Build history of the part. All positions in model axes, mm. A direction names the side the tool comes from. Round coordinates to 2 decimals unless told otherwise and drop trailing zeros. Order: outer loops, then holes, each group sorted by start corner. A loop starts at its lowest first (then second) coordinate and runs counter-clockwise, first axis right, second up. Notation, with made-up numbers: (79, 4.25) - (125, 4.25) arc R17 ccw to (125, 26.25) - close; hole circle Ø2 at (-34.5, -38.75). An arc over 180 degrees is marked (long way). Write each question's results on one line, items separated by ' | '. Start each with the question number.
```python
from build123d import *

# Parameters (mm, degrees)
BOSS_EXTRUDE1_DEPTH = 30
CUT_EXTRUDE3_DEPTH  = 28
SKETCH5_R           = 7.5
CUT_EXTRUDE5_DEPTH  = 4


with BuildPart() as part:
    # Sketch1 → Boss-Extrude1 (new body)
    with BuildSketch(Plane(origin=(0, 0, 0), x_dir=(1, 0, 0), z_dir=(0, 1, 0))):
        with BuildLine():
            Line((5, 0), (70, 0))
            ThreePointArc((70, 0), (73.535533906, 1.464466094), (75, 5))
            Line((75, 5), (75, 85))
            ThreePointArc((75, 85), (73.535533906, 88.535533906), (70, 90))
            Line((70, 90), (5, 90))
            ThreePointArc((5, 90), (1.464466094, 88.535533906), (0, 85))
            Line((0, 85), (0, 5))
            ThreePointArc((0, 5), (1.464466094, 1.464466094), (5, 0))
        make_face()
    extrude(amount=BOSS_EXTRUDE1_DEPTH)

    # Sketch3 → Cut-Extrude3 (cut)
    with BuildSketch(Plane(origin=(0, 0, 0), x_dir=(-1, 0, 0), z_dir=(0, -1, 0))):
        with BuildLine():
            Line((-7.5, 2.5), (-67.5, 2.5))
            ThreePointArc((-67.5, 2.5), (-71.035533906, 3.964466094), (-72.5, 7.5))
            Line((-72.5, 7.5), (-72.5, 82.5))
            ThreePointArc((-72.5, 82.5), (-71.035533906, 86.035533906), (-67.5, 87.5))
            Line((-67.5, 87.5), (-7.5, 87.5))
            ThreePointArc((-7.5, 87.5), (-3.964466094, 86.035533906), (-2.5, 82.5))
            Line((-2.5, 82.5), (-2.5, 7.5))
            ThreePointArc((-2.5, 7.5), (-3.964466094, 3.964466094), (-7.5, 2.5))
        make_face()
    extrude(amount=-CUT_EXTRUDE3_DEPTH, mode=Mode.SUBTRACT)

    # Sketch5 → Cut-Extrude5 (cut)
    with BuildSketch(Plane(origin=(75, 0, 0), x_dir=(0, 0, -1), z_dir=(1, 0, 0))):
        with Locations((35, 15)):
            Circle(SKETCH5_R)
    extrude(amount=-CUT_EXTRUDE5_DEPTH, mode=Mode.SUBTRACT)


solid = part.part
```
1. Wall check: line 1 (X direction, y = 16.75, z = -67); line 2 (Z direction, x = 62, y = 8.25); line 3 (Y direction, x = 73.6, z = -35). Give the ranges that are in metal, low to high. Write a range as from..to.
2. Cut at C-C (x = 61.5). List the corners of the cut face in (y, z), plus the area to 3 significant figures.
3. Cut at B-B (y = 15). List the corners of the cut face in (x, z), plus the area to 4 significant figures.
4. Cut at A-A (z = -35). List the corners of the cut face in (x, y), plus the area to 4 significant figures.
5. Mould opens along X. For faces 4 (the face through (1, 15, -2)), 5 (the face through (71, 13.8, -3.93)), 6 (the face through (73, 15, -1)) say: pulls with the +X half, pulls with the -X half, needs draft (parallel to the pull), parting line crosses it, or undercut.
6. 3-axis set-ups, long thin cutter, end or side, ignore diameter. For faces 1 (the face through (37, 15, 0)), 2 (the face through (37, 14, -2.5)), 3 (the face through (73.8, 20.1, -29.5)): which of +Z, -Z, +X, -X, +Y, -Y reach the whole face in a straight line?
7. Cut at D-D (z = -64.5). List the corners of the cut face in (x, y), plus the area to 3 significant figures.
8. Flat gauge pin, fed straight in: pin 1 Ø6 at (x, z) = (40, -45.5) entering from -Y. Where does the tip first touch, or does it go through?
A:
1) line 1: x = 0..2.5, 72.5..75 | line 2: z = -90..-87.5, -2.5..0 | line 3: y = 0..7.5, 22.5..30
2) outline: (0, -90) - (30, -90) - (30, 0) - (0, 0) - (0, -2.5) - (28, -2.5) - (28, -87.5) - (0, -87.5) - close | area: 320 mm^2
3) outline: (0, -85) arc R5 ccw to (5, -90) - (70, -90) arc R5 ccw to (75, -85) - (75, -42.5) - (72.5, -42.5) - (72.5, -82.5) arc R5 cw to (67.5, -87.5) - (7.5, -87.5) arc R5 cw to (2.5, -82.5) - (2.5, -7.5) arc R5 cw to (7.5, -2.5) - (67.5, -2.5) arc R5 cw to (72.5, -7.5) - (72.5, -27.5) - (75, -27.5) - (75, -5) arc R5 ccw to (70, 0) - (5, 0) arc R5 ccw to (0, -5) - close | area: 762.5 mm^2
4) outline: (0, 0) - (2.5, 0) - (2.5, 28) - (72.5, 28) - (72.5, 22.5) - (75, 22.5) - (75, 30) - (0, 30) - close; (72.5, 0) - (75, 0) - (75, 7.5) - (72.5, 7.5) - close | area: 252.5 mm^2
5) face 4: pulls with the -X half | face 5: undercut | face 6: pulls with the +X half
6) face 1: +Z, +X, -X, +Y, -Y | face 2: -Y | face 3: +X
7) outline: (0, 0) - (2.5, 0) - (2.5, 28) - (72.5, 28) - (72.5, 0) - (75, 0) - (75, 30) - (0, 30) - close | area: 290 mm^2
8) pin 1: stops at y = 28
